```python
from build123d import *

# Parameters (mm, degrees)
SKETCH1_R           = 7.5
BOSS_EXTRUDE1_DEPTH = 16.5
FILLET1_R           = 0.5
SKETCH2_R           = 2.750419987
CUT_EXTRUDE1_DEPTH  = 5
SKETCH3_R           = 7.5
SKETCH3_R_2         = 6.914968151
CUT_EXTRUDE2_DEPTH  = 1
SKETCH4_R           = 1
CUT_EXTRUDE3_DEPTH  = 17.5
SKETCH5_W           = 3.999641176
SKETCH5_H           = 1
CUT_EXTRUDE4_DEPTH  = 0.5


with BuildPart() as part:
    # Sketch1 → Boss-Extrude1 (new body)
    with BuildSketch(Plane(origin=(0, 0, 0), x_dir=(1, 0, 0), z_dir=(0, 1, 0))):
        Circle(SKETCH1_R)
    extrude(amount=BOSS_EXTRUDE1_DEPTH)

    # Fillet1
    fillet1_edges = [part.edges().sort_by_distance(p)[0] for p in [
        (-7.5, 16.5, 0),
    ]]
    fillet(fillet1_edges, radius=FILLET1_R)

    # Sketch2 → Cut-Extrude1 (cut)
    with BuildSketch(Plane.XZ):
        Circle(SKETCH2_R)
    extrude(amount=-CUT_EXTRUDE1_DEPTH, mode=Mode.SUBTRACT)

    # Sketch3 → Cut-Extrude2 (cut)
    with BuildSketch(Plane.XZ):
        Circle(SKETCH3_R)
        Circle(SKETCH3_R_2, mode=Mode.SUBTRACT)
    extrude(amount=-CUT_EXTRUDE2_DEPTH, mode=Mode.SUBTRACT)

    # Sketch4 → Cut-Extrude3 (cut, through all)
    with BuildSketch(Plane(origin=(0, 16.5, 0), x_dir=(1, 0, 0), z_dir=(0, 1, 0))):
        with Locations((1.198920421, -7.909651688)):
            Circle(SKETCH4_R)
        with Locations((-4.165799776, -6.829795914)):
            Circle(SKETCH4_R)
        with Locations((-7.58129596, -2.554202727)):
            Circle(SKETCH4_R)
        with Locations((-7.449419507, 2.916530302)):
            Circle(SKETCH4_R)
        with Locations((-3.831876876, 7.02258639)):
            Circle(SKETCH4_R)
        with Locations((1.578643531, 7.842696258)):
            Circle(SKETCH4_R)
        with Locations((6.250499086, 4.993121386)):
            Circle(SKETCH4_R)
        with Locations((7.997676652, -0.192790476)):
            Circle(SKETCH4_R)
        with Locations((6.002652428, -5.288493531)):
            Circle(SKETCH4_R)
    extrude(amount=-CUT_EXTRUDE3_DEPTH, mode=Mode.SUBTRACT)

    # Sketch5 → Cut-Extrude4 (cut)
    with BuildSketch(Plane(origin=(0, 16.5, 0), x_dir=(1, 0, 0), z_dir=(0, 1, 0))):
        with Locations((-5.951382342, 0)):
            Rectangle(SKETCH5_W, SKETCH5_H)
    extrude(amount=-CUT_EXTRUDE4_DEPTH, mode=Mode.SUBTRACT)


solid = part.part
```
Work out the finished part from the listing and answer in its coordinate system (mm). A direction names the side the tool comes from. Coordinates: 2 decimals unless noted, no trailing zeros. Order: outer loops, then holes, each group sorted by start corner. A loop starts at its lowest first (then second) coordinate and runs counter-clockwise, first axis right, second up. Notation, with made-up numbers: M -10,-2.75 L 15,-2.75 A24 ccw 15,25.25 Z; hole C 57,8.25 d5. An arc over 180 degrees is marked long. Use CSV: the item, a comma, the result in double quotes.
1) Section B-B on y = 13 is taken. Write down the section's boundary in (x, z) (1 decimal).
Worked out:
outline,"M -7.3,1.6 A7.5 ccw -7.2,-1.9 A1 cw -6.6,-3.5 A7.5 ccw -4.3,-6.1 A1 cw -2.8,-6.9 A7.5 ccw 0.6,-7.5 A1 cw 2.3,-7.1 A7.5 ccw 5.3,-5.3 A1 cw 6.3,-4 A7.5 ccw 7.5,-0.7 A1 cw 7.4,1 A7.5 ccw 6.1,4.3 A1 cw 5,5.6 A7.5 ccw 1.9,7.2 A1 cw 0.3,7.5 A7.5 ccw -3.2,6.8 A1 cw -4.6,5.9 A7.5 ccw -6.8,3.2 A1 cw Z"
2) Determine the mould class of faces 1 (the face through (1.06, 8.86, 6.92)), 2 (the face through (-6.523, 8.859, -2.539)), 3 (the face through (7, 1, -2)) for opening direction Z: released by +Z, released by -Z, zero draft, split by the parting line, or undercut.
Worked out:
face 1,"released by +Z"
face 2,"undercut"
face 3,"zero draft"
3) Section A-A on x = 0 is taken. Write down the section's boundary in (y, z).
Worked out:
outline,"M 0,-6.91 L 1,-6.91 L 1,-7.5 L 16,-7.5 A0.5 ccw 16.5,-7 L 16.5,7 A0.5 ccw 16,7.5 L 1,7.5 L 1,6.91 L 0,6.91 L 0,2.75 L 5,2.75 L 5,-2.75 L 0,-2.75 Z"
4) Consider line 1 (Z direction, x = 0, y = 1.9); line 2 (X direction, y = 1.5, z = 1.5); line 3 (Y direction, x = 0.5, z = 1.75). Determine where each line is inside the solid, lowest interval first. Write a range as [from, to].
Worked out:
line 1,"z = [-7.5, -2.75], [2.75, 7.5]"
line 2,"x = [-7.35, -2.31], [2.31, 7.35]"
line 3,"y = [5, 16.5]"
5) Flat-ended cylindrical pins translate along their axes: pin 1 Ø6 at (y, z) = (2.5, -5.5) entering from -X; pin 2 Ø0.8 at (x, z) = (-6, 0) entering from +Y; pin 3 Ø2 at (y, z) = (4, -5.5) entering from -X. Find the tip coordinate at first contact, or state that the pin passes through.
Worked out:
pin 1,"stops at x = -6.63"
pin 2,"stops at y = 16"
pin 3,"stops at x = -6"
6) For faces 4 (the face through (7, 8.86, 0.15)), 5 (the face through (-6, 16, 0)), 6 (the face through (6.596, 0.493, 2.077)), determine the directions among +Z, -Z, +X, -X, +Y, -Y from which every point of the face is accessible in a straight line to the end or side of a thin tool.
Worked out:
face 4,"+X, +Y, -Y"
face 5,"-X, +Y"
face 6,"-Y"
